Autodesk Inventor part; units mm, degrees
ref_plane "YZ Plane" through (0, 0, 0) normal (1, 0, 0) x (0, 1, 0)
ref_plane "XZ Plane" through (0, 0, 0) normal (0, 1, 0) x (-1, 0, 0)
ref_plane "XY Plane" through (0, 0, 0) normal (0, 0, 1) x (1, 0, 0)
sketch "Sketch2" plane through (0, 0, 0) normal (0, 1, 0) x (-1, 0, 0)
  line L0 (0, 0) -> (-337, 0)
  line L1 (-337, 0) -> (-337, -193)
  line L2 (-337, -193) -> (0, -193)
  line L3 (0, -193) -> (0, 0)
  dimension "d3" = 337
  dimension "d4" = 193
extrude "Plate1" add sketch "Sketch2" along normal blind 1.2
sketch "Sketch3" plane through (337, 2.4, 1.2) normal (0, 0, 1) x (1, 0, 0)
  line L0 (-337, 0) -> (0, 0)
  line L1 (0, 0) -> (0, 27.9)
  line L2 (0, 27.9) -> (-337, 27.9)
  line L3 (-337, 27.9) -> (-337, 0)
edge flange "Flange1" height 30.3 angle 90 thickness 1.2 bend radius 1.2 thickness toward (0, 0, 1) relief tear relief width 1.2 relief depth 0.6 edges at (168.5, 1.2, 0) wall of the first edge with corners at (0, 2.4, 1.2) (337, 2.4, 1.2) (337, 30.3, 1.2) (0, 30.3, 1.2)
bend "Bend1"
corner "Corner1"
sketch "Sketch4" plane through (337, 30.3, 1.2) normal (0, 0, -1) x (-1, 0, 0)
  line L0 (337, 0) -> (337, -27.9)
  line L1 (0, 0) -> (0, -27.9)
  line L2 (337, 0) -> (0, 0)
  point P0 (337, -30.3)
  point P1 (320, -13.95)
  point P2 (168.5, -13.95)
  point P3 (17, -13.95)
  dimension "d16" = 17
  dimension "d17" = 17
  dimension "d18" = 151.5
  dimension "d19" = 13.95
  dimension "d20" = 13.95
  dimension "d21" = 13.95
hole "Hole1" at (17, 16.35, 1.2) at (168.5, 16.35, 1.2) at (320, 16.35, 1.2) direction (0, 0, 1) diameter 5 depth 1.2 tip angle 118
equation "\"d27\" = Thickness"
equation "\"d5\" = Thickness"
equation "\"d6\" = BendReliefWidth"
equation "\"d7\" = BendReliefDepth"
equation "\"d8\" = MinimumRemnant"
equation "\"d9\" = TransitionRadius"
equation "\"d12\" = BendRadius"
equation "\"d13\" = CornerReliefSize"
equation "\"d14\" = GapSize"
equation "\"d15\" = JacobiRadiusSize"
equation "\"BendRadius\" = Thickness"
equation "\"BendReliefWidth\" = Thickness"
equation "\"BendReliefDepth\" = 0.5 * Thickness"
equation "\"CornerReliefSize\" = 4 * Thickness"
equation "\"MinimumRemnant\" = 2 * Thickness"
equation "\"TransitionRadius\" = BendRadius"
equation "\"JacobiRadiusSize\" = BendRadius"
equation "\"GapSize\" = Thickness"
properties part number "Separador" material "Steel ASTM A36"
Work out the finished part from the listing and answer in its coordinate system (mm). A direction names the side the tool comes from. Round coordinates to 2 decimals unless told otherwise and drop trailing zeros. Loops run counter-clockwise (first coordinate to the right, second up) from the corner with the lowest first, then second, coordinate; pieces in that order, holes last.
(1) The part is cut by section A-A, the plane x = 292. Give the vertices of the cut face in (y, z), and give its area (3 significant figures).
Computed values:
outline: (0, -193) - (1.2, -193) - (1.2, 0) arc R1.2 cw to (2.4, 1.2) - (30.3, 1.2) - (30.3, 2.4) - (2.4, 2.4) arc R2.4 ccw to (0, 0) - close
area: 268 mm2
(2) The part is cut by section B-B, the plane z = -43. Give the vertices of the cut face in (x, y), and give its area (3 significant figures).
Computed values:
outline: (0, 0) - (337, 0) - (337, 1.2) - (0, 1.2) - close
area: 404 mm2
(3) For faces 1 (the flat face through (171, 13, 1.2)), 2 (the flat face through (171, 20, 2.4)), determine the directions among +Z, -Z, +X, -X, +Y, -Y from which every point of the face is accessible in a straight line to the end or side of a thin tool.
Computed values:
face 1: -Z, +X, -X, +Y
face 2: +Z, +X, -X, +Y, -Y
(4) Find the intervals of material crossed by L1, parallel to X at y = 16.35, z = 2; L2, parallel to Y at x = 255, z = -23.5; L3, parallel to Z at x = 143, y = 20, in increasing order.
Computed values:
L1: x = 0 to 14.5, 19.5 to 166, 171 to 317.5, 322.5 to 337
L2: y = 0 to 1.2
L3: z = 1.2 to 2.4
(5) Each of these flat-tipped pins is pushed along its axis until it touches: P1, Ø8, axis at x = 279.5, y = 11.5, coming from the -Z side; P2, Ø8, axis at x = 94, z = -151, coming from the +Y side. Where does it stop, or does it pass through?
Computed values:
P1: stops at z = 1.2
P2: stops at y = 1.2
